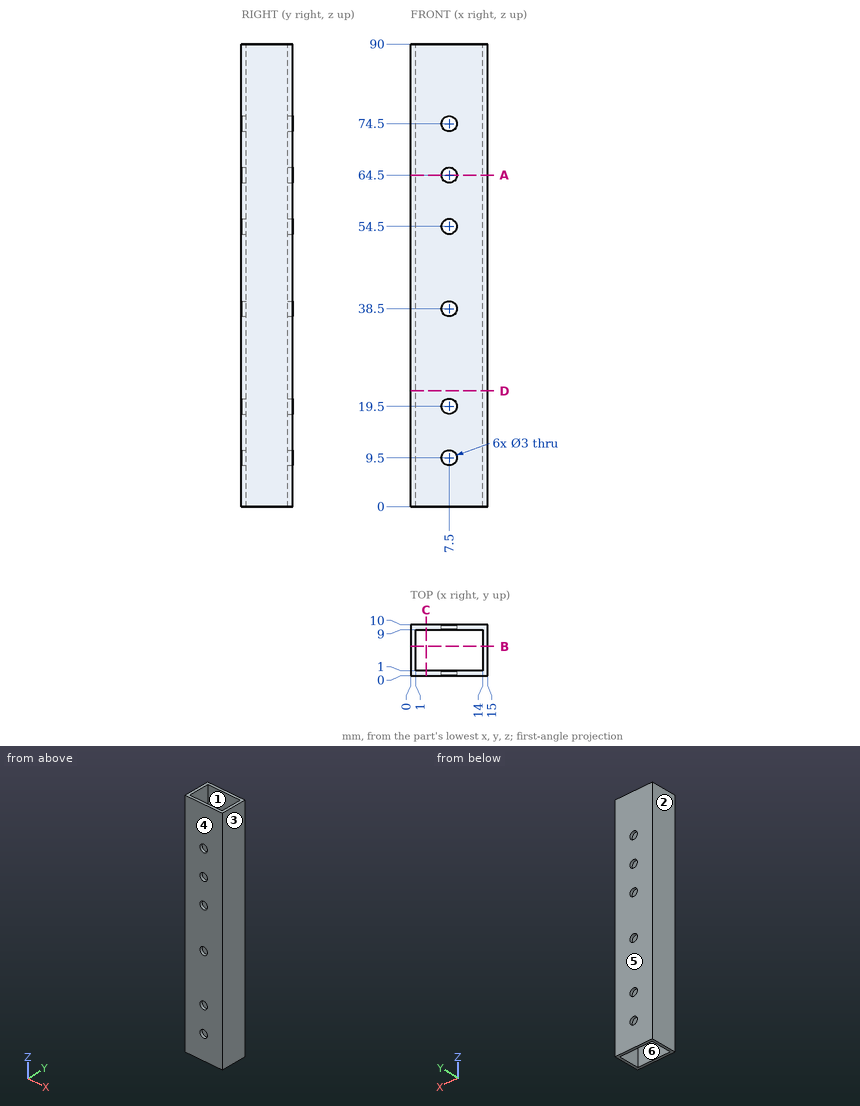
For this review, use the dimensioned drawing (mm, ordinates from the lowest corner) and the shaded views. A direction names the side the tool comes from. Coordinates: 2 decimals unless noted, no trailing zeros. Order: outer loops, then holes, each group sorted by start corner. A loop starts at its lowest first (then second) coordinate and runs counter-clockwise, first axis right, second up. Notation, with made-up numbers: (4.25, 28.25) - (19.25, 28.25) arc R17 cw to (19.25, 46.25) - close; hole circle Ø5 at (34, -7). An arc over 180 degrees is marked (long way). Answer in a Markdown table with one row per item.
(1) Consider section A-A on z = 64.5. State the section outline as (x, y) points, plus the area to 3 significant figures.
Checked values:
| item | result |
|---|---|
| outline | (0, 0) - (6, 0) - (6, 1) - (1, 1) - (1, 9) - (6, 9) - (6, 10) - (0, 10) - close; (9, 0) - (15, 0) - (15, 10) - (9, 10) - (9, 9) - (14, 9) - (14, 1) - (9, 1) - close |
| area | 40.0 mm^2 |
(2) Consider section B-B on y = 5.75. State the section outline as (x, z) points, plus the area to 3 significant figures.
Checked values:
| item | result |
|---|---|
| outline | (0, 0) - (1, 0) - (1, 90) - (0, 90) - close; (14, 0) - (15, 0) - (15, 90) - (14, 90) - close |
| area | 180 mm^2 |
(3) The part is to be moulded in two halves that separate along X. For the marked faces 1, 2, 3 and 4, say which applies: released by +X, released by -X, zero draft, split by the parting line, or undercut.
Checked values:
| item | result |
|---|---|
| face 1 | undercut |
| face 2 | released by -X |
| face 3 | released by +X |
| face 4 | zero draft |
(4) Consider section D-D on z = 22.5. State the section outline as (x, y) points, plus the area to 3 significant figures.
Checked values:
| item | result |
|---|---|
| outline | (0, 0) - (15, 0) - (15, 10) - (0, 10) - close; hole (1, 1) - (14, 1) - (14, 9) - (1, 9) - close |
| area | 46.0 mm^2 |
(5) Wall thickness on line 1 along X through (y, z) = (3.75, 26); line 2 along X through (y, z) = (9.35, 19.5); line 3 along Y through (x, z) = (7.5, 70): over which ranges is each line inside the solid? List them lowest first. Write a range as from..to.
Checked values:
| item | result |
|---|---|
| line 1 | 0..1, 14..15 |
| line 2 | 0..6, 9..15 |
| line 3 | 0..1, 9..10 |
(6) Consider section C-C on x = 3. State the section outline as (y, z) points.
Checked values:
| item | result |
|---|---|
| outline | (0, 0) - (1, 0) - (1, 90) - (0, 90) - close; (9, 0) - (10, 0) - (10, 90) - (9, 90) - close |
(7) For the marked faces 5 and 6, list the 3-axis set-ups (+Z, -Z, +X, -X, +Y, -Y) from which the entire face can be reached by the end or side of a thin tool; tool diameter is ignored.
Checked values:
| item | result |
|---|---|
| face 5 | +Z, -Z, +X, -X, +Y |
| face 6 | +Z, -Z |
